from build123d import *

# Parameters (mm, degrees)
SKETCH2_W           = 50
SKETCH2_H           = 25
BOSS_EXTRUDE1_DEPTH = 4
FILLET1_R           = 2.5
SKETCH3_R           = 7.5
CUT_EXTRUDE1_DEPTH  = 2.5
CHAMFER1_SIZE       = 0.5


with BuildPart() as part:
    # Sketch2 → Boss-Extrude1 (new body)
    with BuildSketch(Plane(origin=(0, 0, 0), x_dir=(1, 0, 0), z_dir=(0, 1, 0))):
        Rectangle(SKETCH2_W, SKETCH2_H)
    extrude(amount=BOSS_EXTRUDE1_DEPTH)

    # Fillet1
    fillet1_edges = [part.edges().sort_by_distance(p)[0] for p in [
        (25, 2, 12.5),
        (-25, 2, 12.5),
        (-25, 2, -12.5),
        (25, 2, -12.5),
    ]]
    fillet(fillet1_edges, radius=FILLET1_R)

    # Sketch3 → Cut-Extrude1 (cut)
    with BuildSketch(Plane(origin=(0, 4, 0), x_dir=(1, 0, 0), z_dir=(0, 1, 0))):
        Circle(SKETCH3_R)
    extrude(amount=-CUT_EXTRUDE1_DEPTH, mode=Mode.SUBTRACT)

    # Chamfer1
    chamfer1_edges = [part.edges().sort_by_distance(p)[0] for p in [
        (-7.5, 4, 0),
    ]]
    chamfer(chamfer1_edges, length=CHAMFER1_SIZE)


solid = part.part
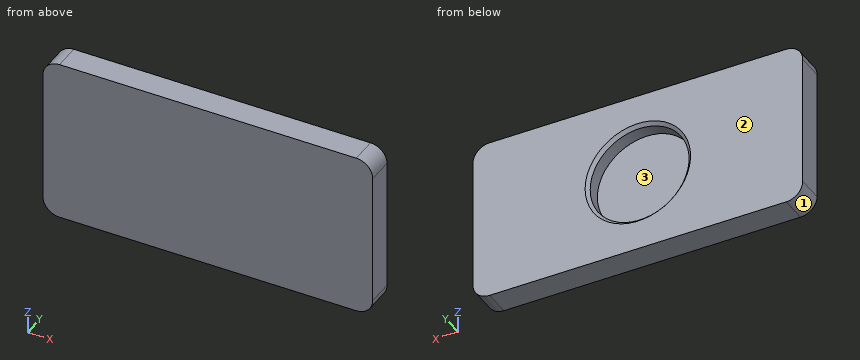
Can you work these out from the model? Positions are in its coordinate system, mm. Face numbers are marked on the shaded views. Coordinates: 2 decimals unless noted, no trailing zeros. Write each loop counter-clockwise with the first axis right and the second up, starting at its lowest first coordinate (ties: lowest second). Pieces come first, ordered by that corner, then holes. Notation, with made-up numbers: (17.25, -34) -> (61.25, -34) arc R32 ccw to (61.25, -3) -> close; hole circle Ø3 at (-35.5, 32). An arc over 180 degrees is marked (long way). Write each question's results on one line, items separated by ' | '. Start each with the question number.
Q1. We'd pull the mould along X, two halves only. Please class the marked faces 1, 2 and 3: +X half, -X half, draft (parallel to the pull), parting line (faces both ways), or undercut.
Q2. Imagine slicing it at A-A (z = 0). Write out the boundary of the cut face in (x, y), then the cut area to 3 significant figures.
Q3. I'm going to push a flat-ended pin straight in: pin 1 (7.5 mm diameter, centred on x = -2.5, z = 0.5, fed in from +Y). Where does the tip first touch, or does it pass through?
Q4. If I drill on probe 1 along Z at (x, y) = (0, 2.3); probe 2 along X at (y, z) = (2.5, 0); probe 3 along X at (y, z) = (2.05, 5.25), over which ranges is the centre line in solid material (lowest first)?
Q5. Imagine slicing it at B-B (x = 0). Write out the boundary of the cut face in (y, z).
Taken from the geometry:
1) face 1: -X half | face 2: draft | face 3: undercut
2) outline: (-25, 0) -> (25, 0) -> (25, 4) -> (8, 4) -> (7.5, 3.5) -> (7.5, 1.5) -> (-7.5, 1.5) -> (-7.5, 3.5) -> (-8, 4) -> (-25, 4) -> close | area: 162 mm^2
3) pin 1: stops at y = 1.5
4) probe 1: z = -12.5 to -7.5, 7.5 to 12.5 | probe 2: x = -25 to -7.5, 7.5 to 25 | probe 3: x = -25 to -5.36, 5.36 to 25
5) outline: (0, -12.5) -> (4, -12.5) -> (4, -8) -> (3.5, -7.5) -> (1.5, -7.5) -> (1.5, 7.5) -> (3.5, 7.5) -> (4, 8) -> (4, 12.5) -> (0, 12.5) -> close
